Source: CAD feature listing. Evaluate the final solid. Frame: model axes, mm. A direction names the side the tool comes from. Round coordinates to 2 decimals unless told otherwise and drop trailing zeros. Order: outer loops, then holes, each group sorted by start corner. A loop starts at its lowest first (then second) coordinate and runs counter-clockwise, first axis right, second up. Notation, with made-up numbers: (-20, 82) -> (22, 82) arc R37 cw to (22, 118) -> close; hole circle Ø8 at (66.25, 81.5). An arc over 180 degrees is marked (long way). One line per item, written item: value. Start each with the question number.
1) Section C-C (y = 0.6). State how many separate pieces and enclosed holes the cut face has, and give its area (3 significant figures).
2) Ray query, L1, parallel to X at y = 1.7, z = 23; L2, parallel to X at y = 2.55, z = -83. Return the intervals inside material, ascending.
3) Pin query (flat end, axial travel): P1, Ø1, axis at x = -60, y = 2.5, coming from the -Z side; P2, Ø1.2, axis at y = 2.5, z = -15, coming from the -X side; P3, Ø1.5, axis at y = 1, z = 60, coming from the +X side. Return the tip coordinate at first contact, or that it passes through.
4) Mould query, pull axis X, two halves, no side actions, for faces 1 (the face through (-83.775, 1.972, -71.047)), 2 (the face through (77.5, 2, -1)), 3 (the face through (-67.5, 2, 1)). Classes: pulls with the +X half, pulls with the -X half, needs draft (parallel to the pull), parting line crosses it, or undercut.
5) Section B-B (z = 22.5). Return the cut outline in (x, y), and give its area (3 significant figures).
6) Reachability of faces 4 (the face through (67.5, 2, 1)), 5 (the face through (-83.953, 1.972, 71.225)), 6 (the face through (83.775, 1.972, 71.047)), 7 (the face through (1, 2, 77.5)), 8 (the face through (-1, 2, -77.5)) from +Z, -Z, +X, -X, +Y, -Y: full face, straight path, thin tool, end or side. Return the list, or none.
7) Section A-A (x = 28). Return the cut outline in (y, z), and give its area (3 significant figures).
```python
from build123d import *

# Parameters (mm, degrees)
SKETCH_1_R      = 1.6
SKETCH_1_W      = 135
SKETCH_1_H      = 135
EXTRUDE_1_DEPTH = 4


with BuildPart() as part:
    # 草图1 → 凸台-拉伸1 (new body)
    with BuildSketch(Plane(origin=(0, 0, 0), x_dir=(1, 0, 0), z_dir=(0, 1, 0))):
        Polygon((90.227922061, 77.5), (77.5, 64.772077939), (77.5, -64.772077939), (90.227922061, -77.5), (77.5, -90.227922061), (64.772077939, -77.5), (-64.772077939, -77.5), (-77.5, -90.227922061), (-90.227922061, -77.5), (-77.5, -64.772077939), (-77.5, 64.772077939), (-90.227922061, 77.5), (-77.5, 90.227922061), (-64.772077939, 77.5), (64.772077939, 77.5), (77.5, 90.227922061), align=None)
        with Locations(Location((77.5, 85.985281374, 0), (0, 0, 270))):
            Circle(SKETCH_1_R, mode=Mode.SUBTRACT)
        with Locations(Location((69.014718626, 77.5, 0), (0, 0, 270))):
            Circle(SKETCH_1_R, mode=Mode.SUBTRACT)
        with Locations(Location((77.5, 69.014718626, 0), (0, 0, 270))):
            Circle(SKETCH_1_R, mode=Mode.SUBTRACT)
        with Locations(Location((85.985281374, 77.5, 0), (0, 0, 270))):
            Circle(SKETCH_1_R, mode=Mode.SUBTRACT)
        with Locations(Location((85.985281374, -77.5, 0), (0, 0, 90))):
            Circle(SKETCH_1_R, mode=Mode.SUBTRACT)
        with Locations(Location((77.5, -69.014718626, 0), (0, 0, 90))):
            Circle(SKETCH_1_R, mode=Mode.SUBTRACT)
        with Locations(Location((69.014718626, -77.5, 0), (0, 0, 90))):
            Circle(SKETCH_1_R, mode=Mode.SUBTRACT)
        with Locations(Location((77.5, -85.985281374, 0), (0, 0, 90))):
            Circle(SKETCH_1_R, mode=Mode.SUBTRACT)
        with Locations(Location((-77.5, -85.985281374, 0), (0, 0, 270))):
            Circle(SKETCH_1_R, mode=Mode.SUBTRACT)
        with Locations(Location((-69.014718626, -77.5, 0), (0, 0, 270))):
            Circle(SKETCH_1_R, mode=Mode.SUBTRACT)
        with Locations(Location((-77.5, -69.014718626, 0), (0, 0, 270))):
            Circle(SKETCH_1_R, mode=Mode.SUBTRACT)
        with Locations(Location((-85.985281374, -77.5, 0), (0, 0, 270))):
            Circle(SKETCH_1_R, mode=Mode.SUBTRACT)
        with Locations(Location((-85.985281374, 77.5, 0), (0, 0, 90))):
            Circle(SKETCH_1_R, mode=Mode.SUBTRACT)
        with Locations(Location((-77.5, 69.014718626, 0), (0, 0, 90))):
            Circle(SKETCH_1_R, mode=Mode.SUBTRACT)
        with Locations(Location((-69.014718626, 77.5, 0), (0, 0, 90))):
            Circle(SKETCH_1_R, mode=Mode.SUBTRACT)
        with Locations(Location((-77.5, 85.985281374, 0), (0, 0, 90))):
            Circle(SKETCH_1_R, mode=Mode.SUBTRACT)
        Rectangle(SKETCH_1_W, SKETCH_1_H, mode=Mode.SUBTRACT)
    extrude(amount=EXTRUDE_1_DEPTH)


solid = part.part
```
Findings:
1. separate pieces: 1
1. enclosed holes: 17
1. area: 6,640 mm2
2. L1: -77.5 to -67.5, 67.5 to 77.5
2. L2: -84.73 to -70.27, 70.27 to 84.73
3. P1: z = -77.5
3. P2: x = -77.5
3. P3: x = 77.5
4. face 1: pulls with the -X half
4. face 2: pulls with the +X half
4. face 3: undercut
5. outline: (-77.5, 0) -> (-67.5, 0) -> (-67.5, 4) -> (-77.5, 4) -> close; (67.5, 0) -> (77.5, 0) -> (77.5, 4) -> (67.5, 4) -> close
5. area: 80.0 mm2
6. face 4: +Y, -Y
6. face 5: -X, +Y, -Y
6. face 6: +X, +Y, -Y
6. face 7: +Z, +Y, -Y
6. face 8: -Z, +Y, -Y
7. outline: (0, -77.5) -> (4, -77.5) -> (4, -67.5) -> (0, -67.5) -> close; (0, 67.5) -> (4, 67.5) -> (4, 77.5) -> (0, 77.5) -> close
7. area: 80.0 mm2
